Check sheet for the modelled part. Datum: model origin and axes. Units: mm. Face numbers are marked on the shaded views. Round coordinates to 2 decimals unless told otherwise and drop trailing zeros. Write each loop counter-clockwise with the first axis right and the second up, starting at its lowest first coordinate (ties: lowest second). Pieces come first, ordered by that corner, then holes. Notation, with made-up numbers: M -3,-23 L 31,-23 A28 ccw 31,-4 Z; hole C 36.5,69.25 d7. An arc over 180 degrees is marked long. One line per item, written item: value.
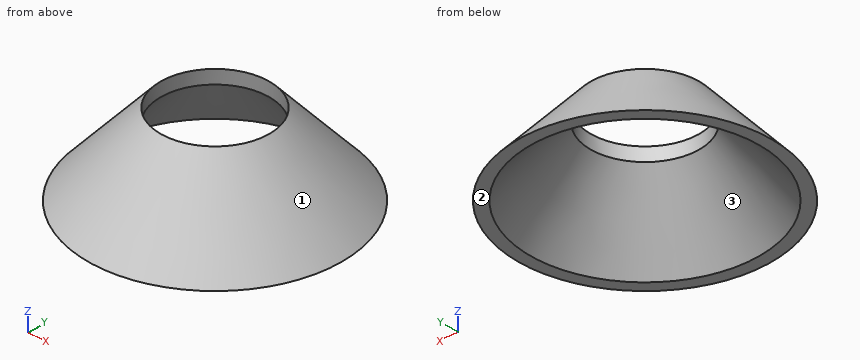
from build123d import *

# Parameters (mm, degrees)
F2_T      = -2.5
F1_FACE_R = 15
F3_DEPTH  = 25


with BuildPart() as f1:
    # F0 (on Front) → F1 (revolve)
    with BuildSketch(Plane.XZ):
        Polygon((0, 0), (0, 22.21225), (-15, 22.21225), (-35, 0), align=None)
    revolve(axis=Axis((0, 0, 30.702899), (0, 0, 1)))

    # F2
    f2_openings = [f1.faces().sort_by_distance(p)[0] for p in [
        (0, 0, 0),
    ]]
    offset(amount=F2_T, openings=f2_openings)

    # F1_face (on face) → F3 (cut)
    with BuildSketch(Plane.XY.offset(22.21225)):
        Circle(F1_FACE_R)
    extrude(amount=-F3_DEPTH, mode=Mode.SUBTRACT)


solid = f1.part
Q1. Sectioned sample at D-D on z = 14.25. Enter the section's corners in (x, y).
Completed:
outline: C 0,0 d44.34; hole C 0,0 d37.61
Q2. Sectioned sample at A-A on y = 0. Enter the section's corners in (x, z), and give its area (3 significant figures).
Completed:
outline: M -35,0 L -31.64,0 L -15,18.48 L -15,22.21 Z; M 15,18.48 L 31.64,0 L 35,0 L 15,22.21 Z
area: 137 mm^2
Q3. Depth check by flat-ended pin: P1, Ø12, axis at x = 13.5, y = 17.5, coming from the +Z side; P2, Ø8, axis at y = -13, z = 17.5, coming from the -X side; P3, Ø6, axis at y = -17.5, z = 6, coming from the +X side. Enter the tip coordinate at first touch or a pass-through.
Completed:
P1: z = 20.99
P2: x = -19.47
P3: x = 27.64
Q4. Scan lines: line 1 (X direction, y = -1.5, z = 11.75); line 2 (X direction, y = 12, z = 5.75); line 3 (Y direction, x = -12, z = 5.25). Record each from-to range of solid material in increasing order. Write a range as [from, to].
Completed:
line 1: [-24.37, -21], [21, 24.37]
line 2: [-27.3, -23.58], [23.58, 27.3]
line 3: [-27.79, -24.08], [24.08, 27.79]
Q5. Sectioned sample at C-C on z = 1.5. Enter the section's corners in (x, y).
Completed:
outline: C 0,0 d67.3; hole C 0,0 d60.57
Q6. Draft check along X on the marked faces 1, 2 and 3. Enter one of: pulls with the +X half, pulls with the -X half, needs draft (parallel to the pull), parting line crosses it, or undercut.
Completed:
face 1: parting line crosses it
face 2: needs draft
face 3: undercut
